The listing builds one solid part. Answer for the finished solid, in the listing's coordinates (mm). A direction names the side the tool comes from. Round coordinates to 2 decimals unless told otherwise and drop trailing zeros. Write each loop counter-clockwise with the first axis right and the second up, starting at its lowest first coordinate (ties: lowest second). Pieces come first, ordered by that corner, then holes.
(1) A cutting plane is placed at D-D, the plane x = 7.5. Give the vertices of the cut face in (y, z), and give its area (3 significant figures).
(2) Find the intervals of material crossed by probe 1 along Y at (x, z) = (-7.5, 2.7); probe 2 along X at (y, z) = (-20.5, 3); probe 3 along Y at (x, z) = (7.5, 5.9), in increasing order.
(3) A cutting plane is placed at A-A, the plane y = 29. Give the vertices of the cut face in (x, z).
(4) Each of these flat-tipped pins is pushed along its axis until it touches: pin 1 Ø1.5 at (x, y) = (19.5, -2) entering from -Z; pin 2 Ø7 at (x, y) = (8, 12.5) entering from +Z. Where does it stop, or does it pass through?
(5) The mould has two halves that part along X. Classify faces 5 (the face through (-5.6, -12.4, 5)), 6 (the face through (-30, -1, 4)), 7 (the face through (0, 1, 0)): +X half, -X half, draft (parallel to the pull), parting line (faces both ways), or undercut.
(6) A cutting plane is placed at C-C, the plane x = -17. Give the vertices of the cut face in (y, z).
(7) A cutting plane is placed at B-B, the plane z = 6. Give the vertices of the cut face in (x, y).
(8) For faces 1 (the face through (14.5, 1, 2)), 2 (the face through (7.4, -14.4, 5)), 3 (the face through (30, -1, 4)), 4 (the face through (-15.9, 1, 6)), determine the directions among +Z, -Z, +X, -X, +Y, -Y from which every point of the face is accessible in a straight line to the end or side of a thin tool.
from build123d import *

# Parameters (mm, degrees)
F0_W     = 60
F0_H     = 80
F0_R     = 4.5
F1_DEPTH = 8
F0_R_2   = 1.6
F2_DEPTH = 5
F3_W     = 1.4
F3_H     = 75
F4_DEPTH = 5
F3_W_2   = 1.6
F3_W_3   = 3.2
F5_DEPTH = 25


with BuildPart() as f1:
    # F0 (on Top) → F1 (new body)
    with BuildSketch(Plane.XY):
        Rectangle(F0_W, F0_H)
        with Locations((-7.5, -12.5)):
            Circle(F0_R, mode=Mode.SUBTRACT)
        with Locations((7.5, -12.5)):
            Circle(F0_R, mode=Mode.SUBTRACT)
        with Locations((-7.5, 12.5)):
            Circle(F0_R, mode=Mode.SUBTRACT)
        with Locations((7.5, 12.5)):
            Circle(F0_R, mode=Mode.SUBTRACT)
    extrude(amount=F1_DEPTH)

    # F0 (on Top) → F2 (join)
    with BuildSketch(Plane.XY):
        with Locations((-7.5, 12.5)):
            Circle(F0_R)
        with Locations((-7.5, 12.5)):
            Circle(F0_R_2, mode=Mode.SUBTRACT)
        with Locations((-7.5, -12.5)):
            Circle(F0_R)
        with Locations((-7.5, -12.5)):
            Circle(F0_R_2, mode=Mode.SUBTRACT)
        with Locations((7.5, -12.5)):
            Circle(F0_R)
        with Locations((7.5, -12.5)):
            Circle(F0_R_2, mode=Mode.SUBTRACT)
        with Locations((7.5, 12.5)):
            Circle(F0_R)
        with Locations((7.5, 12.5)):
            Circle(F0_R_2, mode=Mode.SUBTRACT)
    extrude(amount=F2_DEPTH)

    # F3 (on face) → F4 (cut)
    with BuildSketch(Plane(origin=(0, 0, 0), x_dir=(1, 0, 0), z_dir=(0, 0, -1))):
        with Locations((-19.8, 0)):
            Rectangle(F3_W, F3_H)
        with Locations((-15.2, 0)):
            Rectangle(F3_W, F3_H)
        with Locations((15.2, 0)):
            Rectangle(F3_W, F3_H)
        with Locations((19.8, 0)):
            Rectangle(F3_W, F3_H)
    extrude(amount=-F4_DEPTH, mode=Mode.SUBTRACT)

    # F3 (on face) → F5 (cut)
    with BuildSketch(Plane(origin=(0, 0, 0), x_dir=(1, 0, 0), z_dir=(0, 0, -1))):
        with Locations((-18.3, 0)):
            Rectangle(F3_W_2, F3_H)
        with Locations((-16.7, 0)):
            Rectangle(F3_W_2, F3_H)
        with Locations((17.5, 0)):
            Rectangle(F3_W_3, F3_H)
    extrude(amount=-F5_DEPTH, mode=Mode.SUBTRACT)


solid = f1.part
Solutions:
1. outline: (-40, 0) - (-14.1, 0) - (-14.1, 5) - (-17, 5) - (-17, 8) - (-40, 8) - close; (-10.9, 0) - (10.9, 0) - (10.9, 5) - (8, 5) - (8, 8) - (-8, 8) - (-8, 5) - (-10.9, 5) - close; (14.1, 0) - (40, 0) - (40, 8) - (17, 8) - (17, 5) - (14.1, 5) - close
1. area: 554 mm2
2. probe 1: y = -40 to -14.1, -10.9 to 10.9, 14.1 to 40
2. probe 2: x = -30 to -20.5, -14.5 to 14.5, 20.5 to 30
2. probe 3: y = -40 to -17, -8 to 8, 17 to 40
3. outline: (-30, 0) - (-20.5, 0) - (-20.5, 5) - (-19.1, 5) - (-19.1, 8) - (-30, 8) - close; (-15.9, 5) - (-14.5, 5) - (-14.5, 0) - (14.5, 0) - (14.5, 5) - (15.9, 5) - (15.9, 8) - (-15.9, 8) - close; (19.1, 5) - (20.5, 5) - (20.5, 0) - (30, 0) - (30, 8) - (19.1, 8) - close
4. pin 1: stops at z = 5
4. pin 2: stops at z = 5
5. face 5: undercut
5. face 6: -X half
5. face 7: draft
6. outline: (-40, 0) - (-37.5, 0) - (-37.5, 8) - (-40, 8) - close; (37.5, 0) - (40, 0) - (40, 8) - (37.5, 8) - close
7. outline: (-30, -40) - (30, -40) - (30, 40) - (-30, 40) - close; hole (-19.1, -37.5) - (-15.9, -37.5) - (-15.9, 37.5) - (-19.1, 37.5) - close; hole circle Ø9 at (-7.5, -12.5); hole circle Ø9 at (-7.5, 12.5); hole circle Ø9 at (7.5, -12.5); hole circle Ø9 at (7.5, 12.5); hole (15.9, -37.5) - (19.1, -37.5) - (19.1, 37.5) - (15.9, 37.5) - close
8. face 1: -Z
8. face 2: +Z
8. face 3: +Z, -Z, +X, +Y, -Y
8. face 4: +Z, -Z
